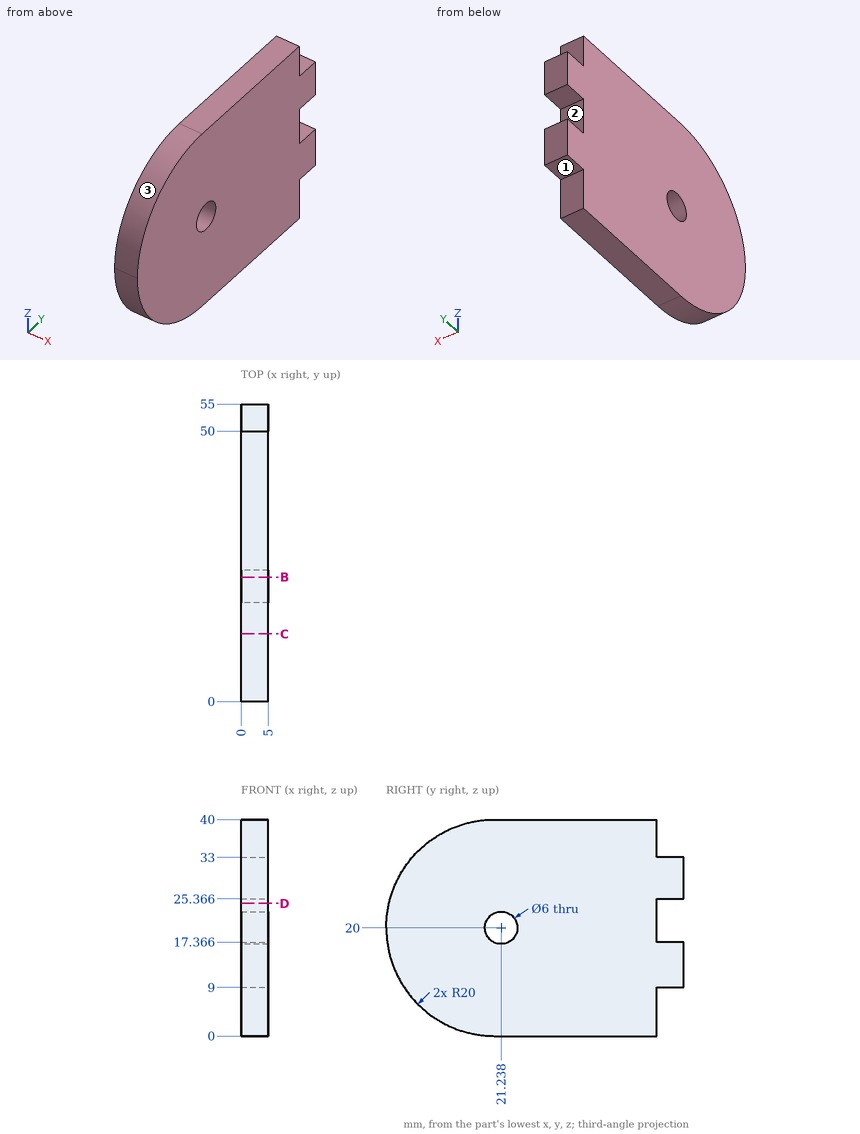
The figure shows three views and two pictorial views of one solid part (mm, origin at its lowest corner). Answer the questions. A direction names the side the tool comes from. Give positions to 0.01 mm unless a question says otherwise; leave off trailing zeros. Order: outer loops, then holes, each group sorted by start corner. A loop starts at its lowest first (then second) coordinate and runs counter-clockwise, first axis right, second up. Notation, with made-up numbers: M 71,-21 L 92,-21 A18 ccw 92,-13 Z; hole C 18.5,31 d8. An arc over 180 degrees is marked long. Return JSON: item names as keys, results as strings.
Q1. Each of these flat-tipped pins is pushed along its axis until it touches: pin 1 (1.5 mm diameter, centred on x = 3.5, z = 35.5, fed in from -Y); pin 2 (1.5 mm diameter, centred on x = 1.5, y = 53, fed in from -Z); pin 3 (7 mm diameter, centred on y = 21.24, z = 20, fed in from -X); pin 4 (1.5 mm diameter, centred on x = 2.5, z = 4.5, fed in from +Y). Where does it stop, or does it pass through?
Answer below:
{"pin 1": "stops at y = 6.49", "pin 2": "stops at z = 9", "pin 3": "stops at x = 0", "pin 4": "stops at y = 50"}
Q2. Find section C-C, the plane y = 12.5. Write down the section's boundary in (x, z), and give its area (3 significant figures).
Answer below:
{"outline": "M 0,1.46 L 5,1.46 L 5,38.54 L 0,38.54 Z", "area": "185 mm^2"}
Q3. Find the intervals of material crossed by line 1 along Y through (x, z) = (2, 20); line 2 along Z through (x, y) = (0.65, 51); line 3 along Y through (x, z) = (1.85, 6.5) (1 decimal), in increasing order. Write a range as [from, to].
Answer below:
{"line 1": "y = [0, 18.24], [24.24, 50]", "line 2": "z = [9, 17.37], [25.37, 33]", "line 3": "y = [5.2, 50]"}
Q4. Find section D-D, the plane z = 24.5. Write down the section's boundary in (x, y).
Answer below:
{"outline": "M 0,0.51 L 5,0.51 L 5,50 L 0,50 Z"}
Q5. Which of the six approach directions +Z, -Z, +X, -X, +Y, -Y give full straight-line access (tool end or side, diameter ignored) to the marked faces 1, 2 and 3?
Answer below:
{"face 1": "-Z, +X, -X, +Y", "face 2": "+X, -X, +Y", "face 3": "+Z, +X, -X, -Y"}
Q6. Find section B-B, the plane y = 23. Write down the section's boundary in (x, z), and give its area (3 significant figures).
Answer below:
{"outline": "M 0,0 L 5,0 L 5,17.57 L 0,17.57 Z; M 0,22.43 L 5,22.43 L 5,40 L 0,40 Z", "area": "176 mm^2"}
